```python
from build123d import *

# Parameters (mm, degrees)
F1_DEPTH = 38.1
F3_DEPTH = 19.05


with BuildPart() as f1:
    # F0 (on Front) → F1 (new body)
    with BuildSketch(Plane.XZ):
        Polygon((-32.421868, 29.878679), (-57.821868, 29.878679), (-57.821868, -33.621321), (43.778132, -33.621321), align=None)
    extrude(amount=F1_DEPTH)

    # F2 (on Front) → F3 (join)
    with BuildSketch(Plane.XZ):
        Polygon((-57.821868, 29.878679), (-57.821868, -33.621321), (72.168774, -33.621321), (72.168774, 4.478679), (43.778132, 29.878679), align=None)
    extrude(amount=F3_DEPTH)


solid = f1.part
```
Input: part model. Units: mm. Frame: model coordinates. A direction names the side the tool comes from. Coordinates: 2 decimals unless noted, no trailing zeros. Loops run counter-clockwise (first coordinate to the right, second up) from the corner with the lowest first, then second, coordinate; pieces in that order, holes last. Notation, with made-up numbers: M 35,63.25 L 93,63.25 A31 cw 93,92.25 Z; hole C 43.25,-36 d5. An arc over 180 degrees is marked long. Answer in a Markdown table with one row per item.
1. Section B-B, the plane x = -23. Output: boundary loops of the cut face in (y, z), then the cut area to 3 significant figures.
Response:
| item | result |
|---|---|
| outline | M -38.1,-33.62 L 0,-33.62 L 0,29.88 L -19.05,29.88 L -19.05,22.03 L -38.1,22.03 Z |
| area | 2,270 mm2 |
2. Section A-A, the plane y = -7.5. Output: boundary loops of the cut face in (x, z), then the cut area to 3 significant figures.
Response:
| item | result |
|---|---|
| outline | M -57.82,-33.62 L 72.17,-33.62 L 72.17,4.48 L 43.78,29.88 L -57.82,29.88 Z |
| area | 7,890 mm2 |
3. Section D-D, the plane y = -32.5. Output: boundary loops of the cut face in (x, z), then the cut area to 3 significant figures.
Response:
| item | result |
|---|---|
| outline | M -57.82,-33.62 L 43.78,-33.62 L -32.42,29.88 L -57.82,29.88 Z |
| area | 4,030 mm2 |
4. Material intervals for line 1 (Y direction, x = 18, z = 9); line 2 (X direction, y = -10, z = 21.5); line 3 (Z direction, x = 38, y = -32), sorted ascending.
Response:
| item | result |
|---|---|
| line 1 | y = -19.05 to 0 |
| line 2 | x = -57.82 to 53.14 |
| line 3 | z = -33.62 to -28.81 |
5. Section C-C, the plane z = -19. Output: boundary loops of the cut face in (x, y).
Response:
| item | result |
|---|---|
| outline | M -57.82,-38.1 L 26.23,-38.1 L 26.23,-19.05 L 72.17,-19.05 L 72.17,0 L -57.82,0 Z |
6. Reachability of faces 1 (the flat face through (31, -19.05, 6)), 2 (the flat face through (6, 0, -1)) from +Z, -Z, +X, -X, +Y, -Y: full face, straight path, thin tool, end or side. Return the list, or none.
Response:
| item | result |
|---|---|
| face 1 | +Z, +X, -Y |
| face 2 | +Z, -Z, +X, -X, +Y |
7. First-contact query: pin 1 (12 mm diameter, centred on y = -33, z = -3.5, fed in from +X); pin 2 (4 mm diameter, centred on x = 10.5, y = -26.5, fed in from +Z); pin 3 (1 mm diameter, centred on x = 52.5, z = -21, fed in from -Y). Flat tips, straight axial feed; report the tip coordinate or a pass-through.
Response:
| item | result |
|---|---|
| pin 1 | stops at x = 14.83 |
| pin 2 | stops at z = -4.22 |
| pin 3 | stops at y = -19.05 |
